Autodesk Inventor part; units mm, degrees
ref_plane "YZ Plane" through (0, 0, 0) normal (1, 0, 0) x (0, 1, 0)
ref_plane "XZ Plane" through (0, 0, 0) normal (0, 1, 0) x (-1, 0, 0)
ref_plane "XY Plane" through (0, 0, 0) normal (0, 0, 1) x (1, 0, 0)
sketch "スケッチ1" plane through (0, 0, 0) normal (1, 0, 0) x (0, 1, 0)
  line L0 (5, 5) -> (-5, 5)
  line L1 (-5, 5) -> (-5, -5)
  line L2 (-5, -5) -> (5, -5)
  line L3 (5, -5) -> (5, 5)
  line L4 (4, 4) -> (-4, 4)
  line L5 (-4, 4) -> (-4, -4)
  line L6 (-4, -4) -> (4, -4)
  line L7 (4, -4) -> (4, 4)
  point P0 (0, 0)
  dimension "d0" = 1
  dimension "d1" = 1
  dimension "d2" = 1
  dimension "d3" = 1
  dimension "d4" = 10
  dimension "d5" = 10
  dimension "d6" = 5
  dimension "d7" = 5
extrude "押し出し1" add sketch "スケッチ1" along normal blind 150
sketch "スケッチ2" plane through (0, -5, 5) normal (0, 0, 1) x (1, 0, 0)
  circle A0 centre (15, 5) radius 1.5
  line L0 (0, 10) -> (0, 0)
  line L1 (0, 0) -> (150, 0)
  circle A1 centre (145, 5) radius 1.5
  line L2 (150, 10) -> (150, 0)
  point P0 (0, 5)
  dimension "d10" = 3
  dimension "d11" = 15
  dimension "d12" = 5
  dimension "d13" = 5
  dimension "d14" = 5
  dimension "d15" = 3
sketch "スケッチ3" plane through (0, -5, -5) normal (0, -1, 0) x (1, 0, 0)
  circle A0 centre (5, 5) radius 1.5
  line L0 (0, 10) -> (0, 0)
  line L1 (0, 0) -> (150, 0)
  point P0 (0, 5)
  dimension "d16" = 3
  dimension "d17" = 5
  dimension "d18" = 5
extrude "押し出し2" cut sketch "スケッチ3" against normal blind 15
extrude "押し出し3" cut sketch "スケッチ2" against normal blind 15
properties part number "backparts1" material "アルミニウム 6061"
For this review, take the finished solid that the model builds, in its own axes (mm). A direction names the side the tool comes from. Coordinates: 2 decimals unless noted, no trailing zeros. Loops run counter-clockwise (first coordinate to the right, second up) from the corner with the lowest first, then second, coordinate; pieces in that order, holes last.
1. Mouldability with a two-part tool opening along Z and no side actions: class faces 3 (the flat face through (74, 0, -5)), 4 (the cylindrical face through (143.5, 0.07, -4.49)), 5 (the flat face through (74, 0, -4)) as +Z half, -Z half, draft (parallel to the pull), parting line (faces both ways), or undercut.
2. Add section A-A, the plane z = 0. Give the boundary of the cut face in (x, y), then the cut area to 3 significant figures.
3. Add section C-C, the plane x = 145. Give the boundary of the cut face in (y, z).
4. For line 1 (Z direction, x = 5, y = 4.4); line 2 (Z direction, x = 112, y = 2), list the stretches that pass through material, from the lowest coordinate up.
5. Add section D-D, the plane x = 109.5. Give the boundary of the cut face in (y, z).
6. Insertion check: P1, Ø1.8, axis at x = 5, z = 0, coming from the -Y side; P2, Ø5, axis at x = 5, z = 0, coming from the +Y side. Each pin has a flat end and moves straight along its axis. Give the tip position at first contact, or say it passes through.
7. Add section B-B, the plane y = 0. Give the boundary of the cut face in (x, z).
8. For faces 1 (the flat face through (74, 4, 0)), 2 (the flat face through (74, 0, 5)), list the 3-axis set-ups (+Z, -Z, +X, -X, +Y, -Y) from which the entire face can be reached by the end or side of a thin tool; tool diameter is ignored.
Result:
1. face 3: -Z half
1. face 4: draft
1. face 5: undercut
2. outline: (0, -5) - (3.5, -5) - (3.5, -4) - (0, -4) - close; (0, 4) - (3.5, 4) - (3.5, 5) - (0, 5) - close; (6.5, -5) - (150, -5) - (150, -4) - (6.5, -4) - close; (6.5, 4) - (150, 4) - (150, 5) - (6.5, 5) - close
2. area: 294 mm2
3. outline: (-5, -5) - (-1.5, -5) - (-1.5, -4) - (-4, -4) - (-4, 4) - (-1.5, 4) - (-1.5, 5) - (-5, 5) - close; (1.5, -5) - (5, -5) - (5, 5) - (1.5, 5) - (1.5, 4) - (4, 4) - (4, -4) - (1.5, -4) - close
4. line 1: z = -5 to -1.5, 1.5 to 5
4. line 2: z = -5 to -4, 4 to 5
5. outline: (-5, -5) - (5, -5) - (5, 5) - (-5, 5) - close; hole (-4, -4) - (4, -4) - (4, 4) - (-4, 4) - close
6. P1: passes through
6. P2: stops at y = 5
7. outline: (0, -5) - (13.5, -5) - (13.5, -4) - (0, -4) - close; (0, 4) - (13.5, 4) - (13.5, 5) - (0, 5) - close; (16.5, -5) - (143.5, -5) - (143.5, -4) - (16.5, -4) - close; (16.5, 4) - (143.5, 4) - (143.5, 5) - (16.5, 5) - close; (146.5, -5) - (150, -5) - (150, -4) - (146.5, -4) - close; (146.5, 4) - (150, 4) - (150, 5) - (146.5, 5) - close
8. face 1: +X, -X
8. face 2: +Z, +X, -X, +Y, -Y
